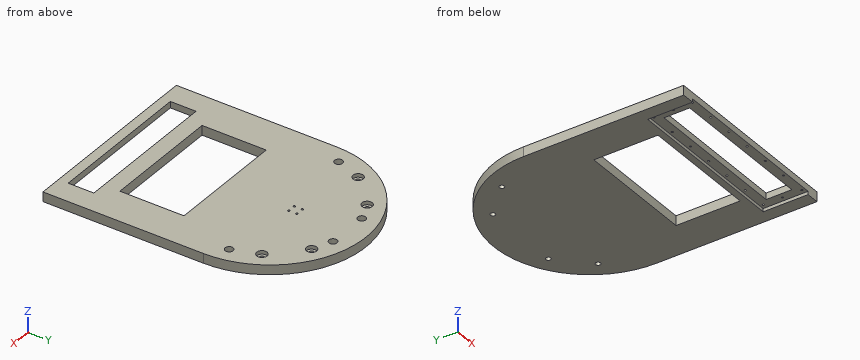
from build123d import *

# Parameters (mm, degrees)
SKETCH_1_R           = 16
EXTRUDE_1_DEPTH      = 30
SKETCH_5_W           = 370
SKETCH_5_H           = 200
CUT_EXTRUDE_3_DEPTH  = 584.86642308
SKETCH_6_W           = 460
SKETCH_6_H           = 80
CUT_EXTRUDE_4_DEPTH  = 100
SKETCH_7_W           = 520
SKETCH_7_H           = 140
CUT_EXTRUDE_5_DEPTH  = 10
SKETCH_10_R          = 12.5
CUT_EXTRUDE_7_DEPTH  = 30
SKETCH_15_R          = 3
CUT_EXTRUDE_12_DEPTH = 10
SKETCH_16_R          = 18.5
SKETCH_16_R_2        = 12.5
EXTRUDE_2_DEPTH      = 5
SKETCH_17_R          = 16
SKETCH_17_R_2        = 7.55
EXTRUDE_4_DEPTH      = 19
EXTRUDE_START        = -10
SKETCH_18_R          = 12.5
EXTRUDE_5_DEPTH      = 10
SKETCH_19_R          = 3.25
CUT_EXTRUDE_13_DEPTH = 10


with BuildPart() as part:
    # 草图1 → 凸台-拉伸1 (new body)
    with BuildSketch(Plane.XY):
        with BuildLine():
            Line((-300, 0), (-300, -500))
            Line((-300, -500), (300, -500))
            Line((300, -500), (300, 0))
            ThreePointArc((300, 0), (0, 300), (-300, 0))
        make_face()
        with Locations((-216.506350946, 125)):
            Circle(SKETCH_1_R, mode=Mode.SUBTRACT)
        with Locations((-125, 216.506350946)):
            Circle(SKETCH_1_R, mode=Mode.SUBTRACT)
        with Locations(Location((125, 216.506350946, 0), (0, 0, 180))):
            Circle(SKETCH_1_R, mode=Mode.SUBTRACT)
        with Locations(Location((216.506350946, 125, 0), (0, 0, 180))):
            Circle(SKETCH_1_R, mode=Mode.SUBTRACT)
    extrude(amount=EXTRUDE_1_DEPTH)

    # 草图5 → 切除-拉伸3 (cut, through all)
    with BuildSketch(Plane.XY.offset(30)):
        with Locations((0, -240)):
            Rectangle(SKETCH_5_W, SKETCH_5_H)
    extrude(amount=-CUT_EXTRUDE_3_DEPTH, mode=Mode.SUBTRACT)

    # 草图6 → 切除-拉伸4 (cut)
    with BuildSketch(Plane.XY.offset(30)):
        with Locations((0, -430)):
            Rectangle(SKETCH_6_W, SKETCH_6_H)
    extrude(amount=-CUT_EXTRUDE_4_DEPTH, mode=Mode.SUBTRACT)

    # 草图7 → 切除-拉伸5 (cut)
    with BuildSketch(Plane(origin=(0, 0, 0), x_dir=(-1, 0, 0), z_dir=(0, 0, -1))):
        with Locations((0, -430)):
            Rectangle(SKETCH_7_W, SKETCH_7_H)
    extrude(amount=-CUT_EXTRUDE_5_DEPTH, mode=Mode.SUBTRACT)

    # 草图10 → 切除-拉伸7 (cut)
    with BuildSketch(Plane.XY.offset(30)):
        with Locations((-246.201938253, 43.412044417)):
            Circle(SKETCH_10_R)
        with Locations((-64.704761276, 241.481456572)):
            Circle(SKETCH_10_R)
        with Locations(Location((246.201938253, 43.412044417, 0), (0, 0, 180))):
            Circle(SKETCH_10_R)
        with Locations(Location((64.704761276, 241.481456572, 0), (0, 0, 180))):
            Circle(SKETCH_10_R)
    extrude(amount=-CUT_EXTRUDE_7_DEPTH, mode=Mode.SUBTRACT)

    # 草图15 → 切除-拉伸12 (cut)
    with BuildSketch(Plane(origin=(0, 0, 10), x_dir=(-1, 0, 0), z_dir=(0, 0, -1))):
        with Locations((0, -370)):
            Circle(SKETCH_15_R)
        with Locations((-82, -370)):
            Circle(SKETCH_15_R)
        with Locations((-164, -370)):
            Circle(SKETCH_15_R)
        with Locations((-246, -370)):
            Circle(SKETCH_15_R)
        with Locations(Location((-246, -490, 0), (0, 0, 180))):
            Circle(SKETCH_15_R)
        with Locations(Location((-164, -490, 0), (0, 0, 180))):
            Circle(SKETCH_15_R)
        with Locations(Location((-82, -490, 0), (0, 0, 180))):
            Circle(SKETCH_15_R)
        with Locations(Location((0, -490, 0), (0, 0, 180))):
            Circle(SKETCH_15_R)
        with Locations((82, -490)):
            Circle(SKETCH_15_R)
        with Locations((164, -490)):
            Circle(SKETCH_15_R)
        with Locations((246, -490)):
            Circle(SKETCH_15_R)
        with Locations(Location((246, -370, 0), (0, 0, 180))):
            Circle(SKETCH_15_R)
        with Locations(Location((164, -370, 0), (0, 0, 180))):
            Circle(SKETCH_15_R)
        with Locations(Location((82, -370, 0), (0, 0, 180))):
            Circle(SKETCH_15_R)
        with Locations((-246, -430)):
            Circle(SKETCH_15_R)
        with Locations((246, -430)):
            Circle(SKETCH_15_R)
    extrude(amount=-CUT_EXTRUDE_12_DEPTH, mode=Mode.SUBTRACT)

    # 草图16 → 凸台-拉伸2 (add)
    # profile 1 of 4: a face of its own
    with BuildSketch(Plane(origin=(0, 0, 0), x_dir=(-1, 0, 0), z_dir=(0, 0, -1))):
        with Locations((-216.506350946, 125)):
            Circle(SKETCH_16_R)
        with Locations((-216.506350946, 125)):
            Circle(SKETCH_16_R_2, mode=Mode.SUBTRACT)
    # profile 2 of 4: a face of its own
    with BuildSketch(Plane(origin=(0, 0, 0), x_dir=(-1, 0, 0), z_dir=(0, 0, -1))):
        with Locations((-125, 216.506350946)):
            Circle(SKETCH_16_R)
        with Locations((-125, 216.506350946)):
            Circle(SKETCH_16_R_2, mode=Mode.SUBTRACT)
    # profile 3 of 4: a face of its own
    with BuildSketch(Plane(origin=(0, 0, 0), x_dir=(-1, 0, 0), z_dir=(0, 0, -1))):
        with Locations((125, 216.506350946)):
            Circle(SKETCH_16_R)
        with Locations(Location((125, 216.506350946, 0), (0, 0, 180))):
            Circle(SKETCH_16_R_2, mode=Mode.SUBTRACT)
    # profile 4 of 4: a face of its own
    with BuildSketch(Plane(origin=(0, 0, 0), x_dir=(-1, 0, 0), z_dir=(0, 0, -1))):
        with Locations((216.506350946, 125)):
            Circle(SKETCH_16_R)
        with Locations(Location((216.506350946, 125, 0), (0, 0, 180))):
            Circle(SKETCH_16_R_2, mode=Mode.SUBTRACT)
    extrude(amount=-EXTRUDE_2_DEPTH)

    # 草图17 → 凸台-拉伸4 (add)
    # profile 1 of 4: a face of its own
    with BuildSketch(Plane(origin=(0, 0, 0), x_dir=(-1, 0, 0), z_dir=(0, 0, -1))):
        with Locations(Location((216.506350946, 125, 0), (0, 0, 180))):
            Circle(SKETCH_17_R)
        with Locations((216.506350946, 125)):
            Circle(SKETCH_17_R_2, mode=Mode.SUBTRACT)
    # profile 2 of 4: a face of its own
    with BuildSketch(Plane(origin=(0, 0, 0), x_dir=(-1, 0, 0), z_dir=(0, 0, -1))):
        with Locations(Location((125, 216.506350946, 0), (0, 0, 180))):
            Circle(SKETCH_17_R)
        with Locations((125, 216.506350946)):
            Circle(SKETCH_17_R_2, mode=Mode.SUBTRACT)
    # profile 3 of 4: a face of its own
    with BuildSketch(Plane(origin=(0, 0, 0), x_dir=(-1, 0, 0), z_dir=(0, 0, -1))):
        with Locations((-125, 216.506350946)):
            Circle(SKETCH_17_R)
        with Locations(Location((-125, 216.506350946, 0), (0, 0, 180))):
            Circle(SKETCH_17_R_2, mode=Mode.SUBTRACT)
    # profile 4 of 4: a face of its own
    with BuildSketch(Plane(origin=(0, 0, 0), x_dir=(-1, 0, 0), z_dir=(0, 0, -1))):
        with Locations((-216.506350946, 125)):
            Circle(SKETCH_17_R)
        with Locations(Location((-216.506350946, 125, 0), (0, 0, 180))):
            Circle(SKETCH_17_R_2, mode=Mode.SUBTRACT)
    extrude(amount=-EXTRUDE_4_DEPTH)

    # 草图18 → 凸台-拉伸5 (add)
    with BuildSketch(Plane(origin=(0, 0, 0), x_dir=(-1, 0, 0), z_dir=(0, 0, -1)).offset(EXTRUDE_START)):
        with Locations((-246.201938253, 43.412044417)):
            Circle(SKETCH_18_R)
        with Locations((-64.704761276, 241.481456572)):
            Circle(SKETCH_18_R)
        with Locations(Location((64.704761276, 241.481456572, 0), (0, 0, 180))):
            Circle(SKETCH_18_R)
        with Locations(Location((246.201938253, 43.412044417, 0), (0, 0, 180))):
            Circle(SKETCH_18_R)
    extrude(amount=EXTRUDE_5_DEPTH)

    # 草图19 → 切除-拉伸13 (cut)
    with BuildSketch(Plane.XY.offset(30)):
        with Locations((-12.375, 92.375)):
            Circle(SKETCH_19_R)
        with Locations((12.375, 92.375)):
            Circle(SKETCH_19_R)
        with Locations((-12.375, 67.625)):
            Circle(SKETCH_19_R)
        with Locations((12.375, 67.625)):
            Circle(SKETCH_19_R)
    extrude(amount=-CUT_EXTRUDE_13_DEPTH, mode=Mode.SUBTRACT)


solid = part.part
Source: CAD feature listing. Evaluate the final solid. Frame: model axes, mm. Coordinates: 2 decimals unless noted, no trailing zeros. Order: outer loops, then holes, each group sorted by start corner. A loop starts at its lowest first (then second) coordinate and runs counter-clockwise, first axis right, second up. Notation, with made-up numbers: M 55,35 L 98,35 A28 cw 98,68 Z; hole C 78,14 d8. An arc over 180 degrees is marked long. Write each question's results on one line, items separated by ' | '. Start each with the question number.
1. Pin query (flat end, axial travel): pin 1 (5 mm diameter, centred on x = 0, y = -370, fed in from -Z); pin 2 (7 mm diameter, centred on x = -246, y = -430, fed in from -Z); pin 3 (5 mm diameter, centred on x = -12.375, y = 67.625, fed in from +Z); pin 4 (13.5 mm diameter, centred on x = 125, y = 216.51, fed in from -Z). Return the tip coordinate at first contact, or that it passes through.
2. Section B-B, the plane z = 25. State how many separate pieces and enclosed holes the cut face has, then the cut area to 3 significant figures.
3. Section A-A, the plane y = -312.5. Return the cut outline in (x, z).
4. Material intervals for L1, parallel to Y at x = -85, z = 28; L2, parallel to X at y = -279, z = 13.75; L3, parallel to Y at x = 205, z = 20, sorted ascending.
5. Section C-C, the plane y = 155. Return the cut outline in (x, z), then the cut area to 3 significant figures.
Solution:
1) pin 1: z = 20 | pin 2: z = 10 | pin 3: z = 20 | pin 4: through
2) separate pieces: 1 | enclosed holes: 14 | area: 325,000 mm²
3) outline: M -300,0 L -185,0 L -185,30 L -300,30 Z; M 185,0 L 300,0 L 300,30 L 185,30 Z
4) L1: -500 to -470, -390 to -340, -140 to 287.71 | L2: -300 to -185, 185 to 300 | L3: -500 to -470, -390 to 113.88, 136.12 to 219.03
5) outline: M -256.86,0 L 256.86,0 L 256.86,30 L -256.86,30 Z | area: 15,400 mm²
